The listing builds one solid part. Answer for the finished solid, in the listing's coordinates (mm). A direction names the side the tool comes from. Coordinates: 2 decimals unless noted, no trailing zeros. Order: outer loops, then holes, each group sorted by start corner. A loop starts at its lowest first (then second) coordinate and runs counter-clockwise, first axis right, second up. Notation, with made-up numbers: M 77,-28 L 92,-28 A19 cw 92,-11 Z; hole C 6,-8 d2. An arc over 180 degrees is marked long. One line per item, written item: value. Start each with the question number.
Q1. The part is cut by section D-D on z = 6.5. Give the vertices of the cut face in (x, y), then the cut area to 3 significant figures.
Q2. Straight lines are drawn through the part: line 1 along Y through (x, z) = (0, 6.85); line 2 along Z through (x, y) = (-1.4, 36); line 3 along X through (y, z) = (35, 8.25). For each, find the intervals that lie inside material, in ascending order. Write a range as [from, to].
Q3. For faces 4 (the flat face through (0, 28, 3)), 5 (the cylindrical face through (-1.5, 0.07, 7.48)), 6 (the flat face through (0, 13, 5)), determine the directions among +Z, -Z, +X, -X, +Y, -Y from which every point of the face is accessible in a straight line to the end or side of a thin tool.
Q4. Determine the mould class of faces 1 (the flat face through (0, 5, 3)), 2 (the flat face through (0, 18, 0)), 3 (the cylindrical face through (0, -3, 7)) for opening direction Z: pulls with the +Z half, pulls with the -Z half, needs draft (parallel to the pull), parting line crosses it, or undercut.
Q5. The part is cut by section B-B on y = 20. Give the vertices of the cut face in (x, z).
Q6. The part is cut by section C-C on x = -2.4. Give the vertices of the cut face in (y, z), then the cut area to 3 significant figures.
Q7. The part is cut by section A-A on x = 0. Give the vertices of the cut face in (y, z), then the cut area to 4 significant figures.
Q8. Each of these flat-tipped pins is pushed along its axis until it touches: pin 1 Ø2.5 at (x, z) = (0, 4.5) entering from +Y; pin 2 Ø0.9 at (x, z) = (-0.5, 4.5) entering from -Y; pin 3 Ø2 at (x, z) = (-1.5, 3) entering from -Y. Where does it stop, or does it pass through?
```python
from build123d import *

# Parameters (mm, degrees)
SCHIZZO2_R                   = 1.5
ESTRUSIONE_ESTRUSIONE1_DEPTH = 9
SCHIZZO5_W                   = 3
SCHIZZO5_H                   = 20.5
SCHIZZO5_H_2                 = 16
TAGLIO_ESTRUSIONE1_DEPTH     = 15


with BuildPart() as part:
    # Schizzo2 → Estrusione-Estrusione1 (new body)
    with BuildSketch(Plane.XY):
        with BuildLine():
            Line((-3, 0), (-3, 35))
            ThreePointArc((-3, 35), (0, 38), (3, 35))
            Line((3, 35), (3, 0))
            ThreePointArc((3, 0), (0, -3), (-3, 0))
        make_face()
        with Locations((0, 35)):
            Circle(SCHIZZO2_R, mode=Mode.SUBTRACT)
        Circle(SCHIZZO2_R, mode=Mode.SUBTRACT)
    extrude(amount=ESTRUSIONE_ESTRUSIONE1_DEPTH)

    # Schizzo5 → Taglio-Estrusione1 (cut)
    with BuildSketch(Plane(origin=(3, 0, 0), x_dir=(0, 0, -1), z_dir=(1, 0, 0))):
        with Locations((-4.5, 27.75)):
            Rectangle(SCHIZZO5_W, SCHIZZO5_H)
        with Locations((-4.5, 5)):
            Rectangle(SCHIZZO5_W, SCHIZZO5_H_2)
    extrude(amount=-TAGLIO_ESTRUSIONE1_DEPTH, mode=Mode.SUBTRACT)


solid = part.part
```
Output:
1. outline: M -3,0 A3 ccw 3,0 L 3,35 A3 ccw -3,35 Z; hole C 0,0 d3; hole C 0,35 d3
1. area: 224 mm^2
2. line 1: y = [-3, -1.5], [1.5, 33.5], [36.5, 38]
2. line 2: z = [0, 3], [6, 9]
2. line 3: x = [-3, -1.5], [1.5, 3]
3. face 4: +X, -X, +Y
3. face 5: +Z, -Z
3. face 6: +X, -X, -Y
4. face 1: undercut
4. face 2: pulls with the -Z half
4. face 3: needs draft
5. outline: M -3,0 L 3,0 L 3,3 L -3,3 Z; M -3,6 L 3,6 L 3,9 L -3,9 Z
6. outline: M -1.8,0 L 36.8,0 L 36.8,3 L 17.5,3 L 17.5,6 L 36.8,6 L 36.8,9 L -1.8,9 L -1.8,6 L 13,6 L 13,3 L -1.8,3 Z
6. area: 245 mm^2
7. outline: M -3,0 L -1.5,0 L -1.5,3 L -3,3 Z; M -3,6 L -1.5,6 L -1.5,9 L -3,9 Z; M 1.5,0 L 33.5,0 L 33.5,3 L 17.5,3 L 17.5,6 L 33.5,6 L 33.5,9 L 1.5,9 L 1.5,6 L 13,6 L 13,3 L 1.5,3 Z; M 36.5,0 L 38,0 L 38,3 L 36.5,3 Z; M 36.5,6 L 38,6 L 38,9 L 36.5,9 Z
7. area: 223.5 mm^2
8. pin 1: stops at y = 17.5
8. pin 2: stops at y = 13
8. pin 3: stops at y = -2.96
